```python
from build123d import *

# Parameters (mm, degrees)
SKETCH1_R           = 0.5
BOSS_EXTRUDE1_DEPTH = 15
FILLET1_R           = 0.75


with BuildPart() as part:
    # Sketch1 → Boss-Extrude1 (new body)
    with BuildSketch(Plane.XY):
        with BuildLine():
            ThreePointArc((9.949874371, -1), (10, 0), (9.949874371, 1))
            ThreePointArc((9.949874371, 1), (7.675986954, 1.279279491), (5.394319042, 1.072996771))
            ThreePointArc((5.394319042, 1.072996771), (5.081337429, 2.104758878), (4.573082868, 3.055636282))
            ThreePointArc((4.573082868, 3.055636282), (6.332329631, 4.523155224), (7.742730421, 6.328516859))
            ThreePointArc((7.742730421, 6.328516859), (7.071067812, 7.071067812), (6.328516859, 7.742730421))
            ThreePointArc((6.328516859, 7.742730421), (4.523155224, 6.332329631), (3.055636282, 4.573082868))
            ThreePointArc((3.055636282, 4.573082868), (2.104758878, 5.081337429), (1.072996771, 5.394319042))
            ThreePointArc((1.072996771, 5.394319042), (1.279279491, 7.675986954), (1, 9.949874371))
            ThreePointArc((1, 9.949874371), (0, 10), (-1, 9.949874371))
            ThreePointArc((-1, 9.949874371), (-1.279279491, 7.675986954), (-1.072996771, 5.394319042))
            ThreePointArc((-1.072996771, 5.394319042), (-2.104758878, 5.081337429), (-3.055636282, 4.573082868))
            ThreePointArc((-3.055636282, 4.573082868), (-4.523155224, 6.332329631), (-6.328516859, 7.742730421))
            ThreePointArc((-6.328516859, 7.742730421), (-7.071067812, 7.071067812), (-7.742730421, 6.328516859))
            ThreePointArc((-7.742730421, 6.328516859), (-6.332329631, 4.523155224), (-4.573082868, 3.055636282))
            ThreePointArc((-4.573082868, 3.055636282), (-5.081337429, 2.104758878), (-5.394319042, 1.072996771))
            ThreePointArc((-5.394319042, 1.072996771), (-7.675986954, 1.279279491), (-9.949874371, 1))
            ThreePointArc((-9.949874371, 1), (-10, 0), (-9.949874371, -1))
            ThreePointArc((-9.949874371, -1), (-7.675986954, -1.279279491), (-5.394319042, -1.072996771))
            ThreePointArc((-5.394319042, -1.072996771), (-5.081337429, -2.104758878), (-4.573082868, -3.055636282))
            ThreePointArc((-4.573082868, -3.055636282), (-6.332329631, -4.523155224), (-7.742730421, -6.328516859))
            ThreePointArc((-7.742730421, -6.328516859), (-7.071067812, -7.071067812), (-6.328516859, -7.742730421))
            ThreePointArc((-6.328516859, -7.742730421), (-4.523155224, -6.332329631), (-3.055636282, -4.573082868))
            ThreePointArc((-3.055636282, -4.573082868), (-2.104758878, -5.081337429), (-1.072996771, -5.394319042))
            ThreePointArc((-1.072996771, -5.394319042), (-1.279279491, -7.675986954), (-1, -9.949874371))
            ThreePointArc((-1, -9.949874371), (0, -10), (1, -9.949874371))
            ThreePointArc((1, -9.949874371), (1.279279491, -7.675986954), (1.072996771, -5.394319042))
            ThreePointArc((1.072996771, -5.394319042), (2.104758878, -5.081337429), (3.055636282, -4.573082868))
            ThreePointArc((3.055636282, -4.573082868), (4.523155224, -6.332329631), (6.328516859, -7.742730421))
            ThreePointArc((6.328516859, -7.742730421), (7.071067812, -7.071067812), (7.742730421, -6.328516859))
            ThreePointArc((7.742730421, -6.328516859), (6.332329631, -4.523155224), (4.573082868, -3.055636282))
            ThreePointArc((4.573082868, -3.055636282), (5.081337429, -2.104758878), (5.394319042, -1.072996771))
            ThreePointArc((5.394319042, -1.072996771), (7.675986954, -1.279279491), (9.949874371, -1))
        make_face()
        Circle(SKETCH1_R, mode=Mode.SUBTRACT)
    extrude(amount=BOSS_EXTRUDE1_DEPTH)

    # Fillet1
    fillet1_edges = [part.edges().sort_by_distance(p)[0] for p in [
        (-3.055636282, 4.573082868, 7.5),
        (-1.072996771, 5.394319042, 7.5),
        (1.072996771, 5.394319042, 7.5),
        (3.055636282, 4.573082868, 7.5),
        (4.573082868, 3.055636282, 7.5),
        (5.394319042, 1.072996771, 7.5),
        (5.394319042, -1.072996771, 7.5),
        (4.573082868, -3.055636282, 7.5),
        (3.055636282, -4.573082868, 7.5),
        (1.072996771, -5.394319042, 7.5),
        (-1.072996771, -5.394319042, 7.5),
        (-3.055636282, -4.573082868, 7.5),
        (-4.573082868, -3.055636282, 7.5),
        (-5.394319042, -1.072996771, 7.5),
        (-5.394319042, 1.072996771, 7.5),
        (-4.573082868, 3.055636282, 7.5),
    ]]
    fillet(fillet1_edges, radius=FILLET1_R)

    # Chamfer1
    # the kernel refuses this chamfer: 0.400753043, 0.25 mm, written as the material it takes off along each edge
    with BuildSketch(Plane(origin=(-1, 9.949874371, -1.002654566), x_dir=(-0.20895056645283513, -0.9779262041580844, 0), z_dir=(0, 0, 1)), Plane(origin=(-6.328516859, -7.742730421, -1.002654566), x_dir=(0.8392486129317811, 0.543747887988617, 0), z_dir=(0, 0, 1)), Plane(origin=(-9.949874371, -1, -1.002654566), x_dir=(0.9779262041580814, -0.20895056645284896, 0), z_dir=(0, 0, 1)), Plane(origin=(-7.742730421, 6.328516859, -1.002654566), x_dir=(0.5437478879886213, -0.8392486129317783, 0), z_dir=(0, 0, 1))) as chamfer1_piece_1:
        with BuildLine():
            Line((0.38673743, 0), (-0.072587978, 0.236060888))
            ThreePointArc((-0.072587978, 0.236060888), (-0.038665519, 0.123154019), (0, 0))
            ThreePointArc((0, 0), (0.200496166, -0.001727616), (0.38673743, 0))
        make_face()
    extrude(amount=17.005309131, mode=Mode.SUBTRACT)
    with BuildSketch(Plane(origin=(1, 9.949874371, -1.000017097), x_dir=(-0.9967308645828112, 0.08079346253256948, 0), z_dir=(0, 0, 1)), Plane(origin=(-7.742730421, -6.328516859, -1.000017097), x_dir=(0.6476655481321507, -0.761924758596727, 0), z_dir=(0, 0, 1)), Plane(origin=(-9.949874371, 1, -1.000017097), x_dir=(-0.0807934625325496, -0.9967308645828128, 0), z_dir=(0, 0, 1)), Plane(origin=(-6.328516859, 7.742730421, -1.000017097), x_dir=(-0.7619247585967629, -0.6476655481321085, 0), z_dir=(0, 0, 1))) as chamfer1_piece_2:
        with BuildLine():
            Line((0.385692125, 0), (-0.072539186, 0.236306293))
            ThreePointArc((-0.072539186, 0.236306293), (-0.038587076, 0.123299359), (0, 0))
            ThreePointArc((0, 0), (0.199968385, -0.001857117), (0.385692125, 0))
        make_face()
    extrude(amount=17.000034195, mode=Mode.SUBTRACT)
    with BuildSketch(Plane(origin=(6.328516859, 7.742730421, -1.002654566), x_dir=(0.7663992656604338, -0.6423645114692652, 0), z_dir=(0, 0, 1)), Plane(origin=(9.949874371, 1, -1.002654566), x_dir=(0.08770581579133363, -0.9961464198983886, 0), z_dir=(0, 0, 1)), Plane(origin=(7.742730421, -6.328516859, -1.002654566), x_dir=(-0.6423645114693267, -0.7663992656603822, 0), z_dir=(0, 0, 1)), Plane(origin=(1, -9.949874371, -1.002654566), x_dir=(-0.9961464198983921, -0.08770581579129355, 0), z_dir=(0, 0, 1))) as chamfer1_piece_3:
        with BuildLine():
            Line((0.246969142, 0), (-0.113667999, -0.36965582))
            ThreePointArc((-0.113667999, -0.36965582), (-0.060580175, -0.19113278), (0, 0))
            ThreePointArc((0, 0), (0.129078874, 0.000760886), (0.246969142, 0))
        make_face()
    extrude(amount=17.005309131, mode=Mode.SUBTRACT)
    with BuildSketch(Plane(origin=(7.742730421, 6.328516859, -1.000017097), x_dir=(-0.538317928460667, -0.8427418394133617, 0), z_dir=(0, 0, 1)), Plane(origin=(9.949874371, -1, -1.000017097), x_dir=(-0.9765567270876431, -0.215260211789988, 0), z_dir=(0, 0, 1)), Plane(origin=(6.328516859, -7.742730421, -1.000017097), x_dir=(-0.8427418394133621, 0.5383179284606663, 0), z_dir=(0, 0, 1)), Plane(origin=(-1, -9.949874371, -1.000017097), x_dir=(-0.21526021179000385, 0.9765567270876397, 0), z_dir=(0, 0, 1))) as chamfer1_piece_4:
        with BuildLine():
            Line((0.247189396, 0), (-0.113183628, -0.368711108))
            ThreePointArc((-0.113183628, -0.368711108), (-0.060457254, -0.190619318), (0, 0))
            ThreePointArc((0, 0), (0.129194415, 0.000705264), (0.247189396, 0))
        make_face()
    extrude(amount=17.000034195, mode=Mode.SUBTRACT)


solid = part.part
```
Geometry check sheet. Reference: the model listing, model coordinates, mm. A direction names the side the tool comes from. Coordinates: 2 decimals unless noted, no trailing zeros. Order: outer loops, then holes, each group sorted by start corner. A loop starts at its lowest first (then second) coordinate and runs counter-clockwise, first axis right, second up. Notation, with made-up numbers: M 0,57 L 31,57 A33 ccw 31,94 Z; hole C 78.25,-9.75 d4. An arc over 180 degrees is marked long. Answer as a JSON object with one key per item and string values.
Q1. Cross-section at A-A on x = 0. Record the cut outline in (y, z), and give its area (3 significant figures).
Results are:
{"outline": "M -10,0 L -0.5,0 L -0.5,15 L -10,15 Z; M 0.5,0 L 10,0 L 10,15 L 0.5,15 Z", "area": "285 mm²"}
Q2. Release check for a two-part mould opening along Y. For faces 6 (the cylindrical face through (-7.11, 7.03, 7.4)), 7 (the cylindrical face through (-0.108, -0.488, 7.395)), 8 (the flat face through (0, 2, 0)) record: released by +Y, released by -Y, zero draft, split by the parting line, or undercut.
Results are:
{"face 6": "released by +Y", "face 7": "undercut", "face 8": "zero draft"}
Q3. Tool access check on faces 1 (the cylindrical face through (-1.275, -7.858, 7.395)), 2 (the cylindrical face through (-6.5, -4.7, 7.4)), 3 (the cylindrical face through (2.099, -5.084, 7.395)), 4 (the cylindrical face through (2.11, 5.08, 7.4)), 5 (the cylindrical face through (5.084, 2.099, 7.395)). Record the directions out of +Z, -Z, +X, -X, +Y, -Y that give a thin tool (end or side, any length) a straight path to the whole face; none if there is none.
Results are:
{"face 1": "+Z, -Z", "face 2": "+Z, -Z, -X", "face 3": "+Z, -Z, -Y", "face 4": "+Z, -Z, +Y", "face 5": "+Z, -Z, +X"}
Q4. Cross-section at C-C on y = 7. Record the cut outline in (x, z).
Results are:
{"outline": "M -7.14,0 L -5.28,0 L -5.28,15 L -7.14,15 Z; M -1.27,0 L 1.27,0 L 1.27,15 L -1.27,15 Z; M 5.28,0 L 7.14,0 L 7.14,15 L 5.28,15 Z"}
Q5. Cross-section at D-D on x = -8.25. Record the cut outline in (y, z), and give its area (3 significant figures).
Results are:
{"outline": "M -1.25,0 L 1.25,0 L 1.25,15 L -1.25,15 Z", "area": "37.6 mm²"}
Q6. Scan lines: line 1 (Y direction, x = 0, z = 3.5); line 2 (Y direction, x = 6.5, z = 2.5); line 3 (Y direction, x = 7.25, z = 3.75). Record each from-to range of solid material in increasing order.
Results are:
{"line 1": "y = -10 to -0.5, 0.5 to 10", "line 2": "y = -7.52 to -4.7, -1.23 to 1.23, 4.7 to 7.58", "line 3": "y = -6.89 to -5.6, -1.28 to 1.28, 5.6 to 6.89"}
Q7. Depth check by flat-ended pin: pin 1 Ø1.5 at (y, z) = (-2.5, 9.5) entering from +X; pin 2 Ø2 at (x, z) = (-1.5, 7) entering from +Y; pin 3 Ø1.5 at (y, z) = (-7.5, 3) entering from -X. Enter the tip coordinate at first touch or a pass-through.
Results are:
{"pin 1": "stops at x = 5.21", "pin 2": "stops at y = 9.99", "pin 3": "stops at x = -7.38"}
